Build history of the part. All positions in model axes, mm. A direction names the side the tool comes from. Give positions to 0.01 mm unless a question says otherwise; leave off trailing zeros. Order: outer loops, then holes, each group sorted by start corner. A loop starts at its lowest first (then second) coordinate and runs counter-clockwise, first axis right, second up. Notation, with made-up numbers: M -26.75,6 L -0.75,6 A11 ccw -0.75,12 Z; hole C 3.5,-11.5 d10. An arc over 180 degrees is marked long. Answer as CSV lines item,"result".
from build123d import *

# Parameters (mm, degrees)
SKETCH2_W                                      = 115.292618629
SKETCH2_H                                      = 134.000000002
BOSS_EXTRUDE2_DEPTH                            = 8
FILLET2_R                                      = 6
SKETCH19_W                                     = 8
SKETCH19_H                                     = 99
BOSS_EXTRUDE3_DEPTH                            = 115.292618629
SKETCH21_W                                     = 135.292618629
SKETCH21_H                                     = 129
SKETCH21_W_2                                   = 115.292618629
SKETCH21_H_2                                   = 99
BOSS_EXTRUDE4_DEPTH                            = 8
FILLET3_R                                      = 5
CUT_EXTRUDE1_DEPTH                             = 4
SKETCH24_W                                     = 115.292618629
SKETCH24_H                                     = 10
BOSS_EXTRUDE5_DEPTH                            = 104
FILLET4_R                                      = 6
SKETCH49_R                                     = 4.43
CUT_EXTRUDE3_DEPTH                             = 8
M2_5_CLEARANCE_HOLE1_D                         = 2.9
CUT_EXTRUDE4_START                             = -8
CUT_EXTRUDE4_DEPTH                             = 8
CHAMFER1_SIZE                                  = 0.9
CSK_FOR_8_FLAT_HEAD_MACHINE_SCREW1_D           = 4.4958
CSK_FOR_8_FLAT_HEAD_MACHINE_SCREW1_DEPTH       = 8
CSK_FOR_8_FLAT_HEAD_MACHINE_SCREW1_CSINK_D     = 10.1713792
CSK_FOR_8_FLAT_HEAD_MACHINE_SCREW1_CSINK_ANGLE = 82
CSK_FOR_8_FLAT_HEAD_MACHINE_SCREW1_TIP         = 1.350674586
SKETCH61_W                                     = 115.292618629
SKETCH61_H                                     = 134.000000002
CUT_EXTRUDE6_DEPTH                             = 65


with BuildPart() as part:
    # Sketch2 → Boss-Extrude2 (new body)
    with BuildSketch(Plane(origin=(0, 0, 0), x_dir=(1, 0, 0), z_dir=(0, 1, 0))):
        with Locations((4.853690686, 42.889279439)):
            Rectangle(SKETCH2_W, SKETCH2_H)
    extrude(amount=BOSS_EXTRUDE2_DEPTH)

    # Fillet2
    fillet2_edges = [part.edges().sort_by_distance(p)[0] for p in [
        (-52.792618629, 4, -109.88927944),
        (62.5, 4, -109.88927944),
    ]]
    fillet(fillet2_edges, radius=FILLET2_R)

    # Sketch19 → Boss-Extrude3 (add)
    with BuildSketch(Plane.ZY.offset(52.792618629)):
        with Locations((28.110720562, 13.5)):
            Rectangle(SKETCH19_W, SKETCH19_H)
    extrude(amount=-BOSS_EXTRUDE3_DEPTH)

    # Sketch21 → Boss-Extrude4 (add)
    with BuildSketch(Plane.XY.offset(32.110720562)):
        with Locations((4.853690685, 8.5)):
            Rectangle(SKETCH21_W, SKETCH21_H)
        with Locations((4.853690686, 13.5)):
            Rectangle(SKETCH21_W_2, SKETCH21_H_2, mode=Mode.SUBTRACT)
    extrude(amount=-BOSS_EXTRUDE4_DEPTH)

    # Fillet3
    fillet3_edges = [part.edges().sort_by_distance(p)[0] for p in [
        (72.5, 73, 28.110720562),
        (72.5, -56, 28.110720562),
        (-62.792618629, -56, 28.110720562),
        (-62.792618629, 73, 28.110720562),
    ]]
    fillet(fillet3_edges, radius=FILLET3_R)

    # Sketch22 → Cut-Extrude1 (cut)
    with BuildSketch(Plane(origin=(0, 0, 24.110720562), x_dir=(-1, 0, 0), z_dir=(0, 0, -1))):
        with BuildLine():
            Line((62.792618629, -51), (62.792618629, 68))
            ThreePointArc((62.792618629, 68), (61.328152535, 71.535533906), (57.792618629, 73))
            Line((57.792618629, 73), (-67.5, 73))
            ThreePointArc((-67.5, 73), (-71.035533906, 71.535533906), (-72.5, 68))
            Line((-72.5, 68), (-72.5, -51))
            ThreePointArc((-72.5, -51), (-71.035533906, -54.535533906), (-67.5, -56))
            Line((-67.5, -56), (57.792618629, -56))
            ThreePointArc((57.792618629, -56), (61.328152535, -54.535533906), (62.792618629, -51))
        make_face()
        with BuildLine():
            Line((57.792618629, 69.75), (-67.5, 69.75))
            ThreePointArc((-67.5, 69.75), (-68.737436867, 69.237436867), (-69.25, 68))
            Line((-69.25, 68), (-69.25, -51))
            ThreePointArc((-69.25, -51), (-68.737436867, -52.237436867), (-67.5, -52.75))
            Line((-67.5, -52.75), (57.792618629, -52.75))
            ThreePointArc((57.792618629, -52.75), (59.030055496, -52.237436867), (59.542618629, -51))
            Line((59.542618629, -51), (59.542618629, 68))
            ThreePointArc((59.542618629, 68), (59.030055496, 69.237436867), (57.792618629, 69.75))
        make_face(mode=Mode.SUBTRACT)
    extrude(amount=-CUT_EXTRUDE1_DEPTH, mode=Mode.SUBTRACT)

    # Sketch24 → Boss-Extrude5 (add)
    with BuildSketch(Plane(origin=(0, 0, 24.110720562), x_dir=(-1, 0, 0), z_dir=(0, 0, -1))):
        with Locations((-4.853690686, 60)):
            Rectangle(SKETCH24_W, SKETCH24_H)
    extrude(amount=BOSS_EXTRUDE5_DEPTH)

    # Fillet4
    fillet4_edges = [part.edges().sort_by_distance(p)[0] for p in [
        (62.5, 60, -79.889279438),
        (-52.792618629, 60, -79.889279438),
    ]]
    fillet(fillet4_edges, radius=FILLET4_R)

    # Sketch49 → Cut-Extrude3 (cut)
    with BuildSketch(Plane.XY.offset(32.110720562)):
        with Locations((4.853690685, 40.159632183)):
            Circle(SKETCH49_R)
    extrude(amount=-CUT_EXTRUDE3_DEPTH, mode=Mode.SUBTRACT)

    # M2.5 Clearance Hole1 (through all)
    with Locations(Plane(origin=(0, 8, 0), x_dir=(1, 0, 0), z_dir=(0, 1, 0))):
        with Locations((-28.27, 101.64), (-7.29, 101.64), (-7.29, 88.14), (-28.27, 88.14)):
            Hole(M2_5_CLEARANCE_HOLE1_D / 2)

    # Sketch60 → Cut-Extrude4 (cut)
    with BuildSketch(Plane(origin=(0, 8, 0), x_dir=(1, 0, 0), z_dir=(0, 1, 0)).offset(CUT_EXTRUDE4_START)):
        with BuildLine():
            Line((-30.27, 103.09), (-26.27, 103.09))
            ThreePointArc((-26.27, 103.09), (-24.82, 101.64), (-26.27, 100.19))
            Line((-26.27, 100.19), (-30.27, 100.19))
            ThreePointArc((-30.27, 100.19), (-31.72, 101.64), (-30.27, 103.09))
        make_face()
        with BuildLine():
            Line((-9.29, 103.09), (-5.29, 103.09))
            ThreePointArc((-5.29, 103.09), (-3.84, 101.64), (-5.29, 100.19))
            Line((-5.29, 100.19), (-9.29, 100.19))
            ThreePointArc((-9.29, 100.19), (-10.74, 101.64), (-9.29, 103.09))
        make_face()
        with BuildLine():
            Line((-30.27, 89.59), (-26.27, 89.59))
            ThreePointArc((-26.27, 89.59), (-24.82, 88.14), (-26.27, 86.69))
            Line((-26.27, 86.69), (-30.27, 86.69))
            ThreePointArc((-30.27, 86.69), (-31.72, 88.14), (-30.27, 89.59))
        make_face()
        with BuildLine():
            Line((-9.29, 89.59), (-5.29, 89.59))
            ThreePointArc((-5.29, 89.59), (-3.84, 88.14), (-5.29, 86.69))
            Line((-5.29, 86.69), (-9.29, 86.69))
            ThreePointArc((-9.29, 86.69), (-10.74, 88.14), (-9.29, 89.59))
        make_face()
    extrude(amount=CUT_EXTRUDE4_DEPTH, mode=Mode.SUBTRACT)

    # Chamfer1
    chamfer1_edges = [part.edges().sort_by_distance(p)[0] for p in [
        (-7.29, 8, -100.19),
        (-3.84, 8, -101.64),
        (-7.29, 8, -103.09),
        (-28.27, 8, -86.69),
        (-24.82, 8, -88.14),
        (-28.27, 8, -89.59),
        (-7.29, 8, -86.69),
        (-3.84, 8, -88.14),
        (-7.29, 8, -89.59),
        (-28.27, 8, -103.09),
        (-31.72, 8, -101.64),
        (-28.27, 8, -100.19),
        (-24.82, 8, -101.64),
        (-10.74, 8, -88.14),
        (-31.72, 8, -88.14),
        (-10.74, 8, -101.64),
    ]]
    chamfer(chamfer1_edges, length=CHAMFER1_SIZE)

    # CSK for #8 Flat Head Machine Screw1
    with Locations(Plane.XY.offset(32.110720562)):
        with Locations((-42.792618629, 60), (52.5, 60), (-42.792618629, 4), (52.5, 4)):
            CounterSinkHole(CSK_FOR_8_FLAT_HEAD_MACHINE_SCREW1_D / 2, CSK_FOR_8_FLAT_HEAD_MACHINE_SCREW1_CSINK_D / 2, depth=CSK_FOR_8_FLAT_HEAD_MACHINE_SCREW1_DEPTH, counter_sink_angle=CSK_FOR_8_FLAT_HEAD_MACHINE_SCREW1_CSINK_ANGLE)
            with Locations((0, 0, -(CSK_FOR_8_FLAT_HEAD_MACHINE_SCREW1_DEPTH + CSK_FOR_8_FLAT_HEAD_MACHINE_SCREW1_TIP / 2))):  # 118° drill point
                Cone(0, CSK_FOR_8_FLAT_HEAD_MACHINE_SCREW1_D / 2, CSK_FOR_8_FLAT_HEAD_MACHINE_SCREW1_TIP, mode=Mode.SUBTRACT)

    # Sketch61 → Cut-Extrude6 (cut)
    with BuildSketch(Plane(origin=(0, 65, 0), x_dir=(1, 0, 0), z_dir=(0, 1, 0))):
        with Locations((4.853690686, 42.889279439)):
            Rectangle(SKETCH61_W, SKETCH61_H)
    extrude(amount=-CUT_EXTRUDE6_DEPTH, mode=Mode.SUBTRACT)


solid = part.part
Item 1: Drop flat-ended pins along their axis: pin 1 (3.5 mm diameter, centred on x = -42.79, y = 4, fed in from +Z); pin 2 (3 mm diameter, centred on y = -0.5, z = 25.5, fed in from +X); pin 3 (3 mm diameter, centred on y = 10.5, z = 27.5, fed in from +X); pin 4 (2 mm diameter, centred on x = -31, z = 25.5, fed in from +Y). Give the stop position or say it passes through.
Geometry says:
pin 1,"passes through"
pin 2,"stops at x = 69.25"
pin 3,"stops at x = 72.5"
pin 4,"stops at y = 69.75"
Item 2: Band-saw the part on C-C (y = 38). Give the cut face in (x, z).
Geometry says:
outline,"M -62.79,28.11 L -59.54,28.11 L -59.54,24.11 L 0.99,24.11 L 0.99,32.11 L -62.79,32.11 Z; M 8.72,24.11 L 69.25,24.11 L 69.25,28.11 L 72.5,28.11 L 72.5,32.11 L 8.72,32.11 Z"
Item 3: 3-axis set-ups, long thin cutter, end or side, ignore diameter. For faces 5 (the flat face through (-59.543, 8, 26)), 6 (the flat face through (69.25, 9, 26)), 7 (the flat face through (10, -53, 28.111)), 8 (the flat face through (4, 69.75, 26)), 9 (the flat face through (6, -52.75, 26)): which of +Z, -Z, +X, -X, +Y, -Y reach the whole face in a straight line?
Geometry says:
face 5,"-Z, -X, +Y, -Y"
face 6,"-Z, +X, +Y, -Y"
face 7,"-Z"
face 8,"-Z, +X, -X, +Y"
face 9,"-Z, +X, -X, -Y"
Item 4: Pull direction X, two halves, no side cores. Call faces 1 (the conical face through (54.258, 5.612, 29.005)), 2 (the conical face through (-40.9, 58.55, 29)), 3 (the cylindrical face through (-61.367, -54.496, 30.083)), 4 (the flat face through (4, -56, 30)): released by +X, released by -X, zero draft, split by the parting line, or undercut.
Geometry says:
face 1,"undercut"
face 2,"undercut"
face 3,"released by -X"
face 4,"zero draft"
Item 5: Band-saw the part on D-D (x = 14). Give the cut face in (y, z), and give its area (3 significant figures).
Geometry says:
outline,"M -56,28.11 L -52.75,28.11 L -52.75,24.11 L 69.75,24.11 L 69.75,28.11 L 73,28.11 L 73,32.11 L -56,32.11 Z"
area,"1,010 mm2"
Item 6: Band-saw the part on B-B (y = 60). Give the cut face in (x, z), and give its area (3 significant figures).
Geometry says:
outline,"M -62.79,28.11 L -59.54,28.11 L -59.54,24.11 L -45.04,24.11 L -45.04,28.85 L -47.88,32.11 L -62.79,32.11 Z; M -40.54,24.11 L 50.25,24.11 L 50.25,28.85 L 47.41,32.11 L -37.71,32.11 L -40.54,28.85 Z; M 54.75,24.11 L 69.25,24.11 L 69.25,28.11 L 72.5,28.11 L 72.5,32.11 L 57.59,32.11 L 54.75,28.85 Z"
area,"966 mm2"
Item 7: Band-saw the part on A-A (x = 52.5). Give the cut face in (y, z).
Geometry says:
outline,"M -56,28.11 L -52.75,28.11 L -52.75,24.11 L 1.75,24.11 L 1.75,28.85 L -1.09,32.11 L -56,32.11 Z; M 6.25,24.11 L 57.75,24.11 L 57.75,28.85 L 54.91,32.11 L 9.09,32.11 L 6.25,28.85 Z; M 62.25,24.11 L 69.75,24.11 L 69.75,28.11 L 73,28.11 L 73,32.11 L 65.09,32.11 L 62.25,28.85 Z"
Item 8: Probe line 1 along X through (y, z) = (60, 26); line 2 along Y through (x, z) = (52.5, 25.8); line 3 along X through (y, z) = (3, 25). List the from-to ranges inside material, lowest first. Write a range as from..to.
Geometry says:
line 1,"x = -59.54..-45.04, -40.54..50.25, 54.75..69.25"
line 2,"y = -52.75..1.75, 6.25..57.75, 62.25..69.75"
line 3,"x = -59.54..-44.81, -40.78..50.49, 54.51..69.25"
